Autodesk Inventor part; units mm, degrees
ref_plane "YZ Plane" through (0, 0, 0) normal (1, 0, 0) x (0, 1, 0)
ref_plane "XZ Plane" through (0, 0, 0) normal (0, 1, 0) x (-1, 0, 0)
ref_plane "XY Plane" through (0, 0, 0) normal (0, 0, 1) x (1, 0, 0)
sketch "スケッチ1" plane through (0, 0, 0) normal (0, 0, 1) x (1, 0, 0)
  point P0 (0, 0)
sketch "スケッチ2" plane through (0, 0, 0) normal (0, 0, 1) x (1, 0, 0)
  line L0 (80, -40) -> (-80, -40)
  line L1 (-80, -40) -> (-80, 40)
  line L2 (-80, 40) -> (80, 40)
  line L3 (80, 40) -> (80, -40)
  line L4 (80, -40) -> (-80, 40) construction
  line L5 (-80, -40) -> (80, 40) construction
  circle A0 centre (-48, -19.5) radius 6.05
  circle A1 centre (48, -19.5) radius 12.55
  circle A2 centre (48, -19.5) radius 17.5
  circle A3 centre (65.5, -19.5) radius 2.05
  circle A4 centre (48, -2) radius 2.05
  circle A5 centre (30.5, -19.5) radius 2.05
  circle A6 centre (48, -37) radius 2.05
  circle A7 centre (-48, -19.5) radius 9
  circle A8 centre (-57, -19.5) radius 1.6
  circle A9 centre (-48, -28.5) radius 1.6
  circle A10 centre (-39, -19.5) radius 1.6
  circle A11 centre (-48, -10.5) radius 1.6
  line L6 (75, 35) -> (-75, 35)
  line L7 (-75, 35) -> (-75, -35)
  line L8 (-75, -35) -> (75, -35)
  line L9 (75, -35) -> (75, 35)
  line L10 (-75, 35) -> (-75, 35) construction
  line L11 (-76.6, 35) -> (-76.6, 35)
  line L12 (-73.4, 35) -> (-73.4, 35)
  arc A12 (-73.4, 35) -> (-76.6, 35) centre (-75, 35) ccw
  arc A13 (-76.6, 35) -> (-73.4, 35) centre (-75, 35) ccw
  line L13 (-75, 35) -> (-75, 35) construction
  line L14 (-75, -35) -> (-75, -35) construction
  line L15 (-73.4, -35) -> (-73.4, -35)
  line L16 (-76.6, -35) -> (-76.6, -35)
  arc A14 (-76.6, -35) -> (-73.4, -35) centre (-75, -35) ccw
  arc A15 (-73.4, -35) -> (-76.6, -35) centre (-75, -35) ccw
  line L17 (-75, -35) -> (-75, -35) construction
  line L18 (75, 35) -> (75, 35) construction
  line L19 (73.4, 35) -> (73.4, 35)
  line L20 (76.6, 35) -> (76.6, 35)
  arc A16 (76.6, 35) -> (73.4, 35) centre (75, 35) ccw
  arc A17 (73.4, 35) -> (76.6, 35) centre (75, 35) ccw
  line L21 (75, 35) -> (75, 35) construction
  line L22 (75, -35) -> (75, -35) construction
  line L23 (76.6, -35) -> (76.6, -35)
  line L24 (73.4, -35) -> (73.4, -35)
  arc A18 (73.4, -35) -> (76.6, -35) centre (75, -35) ccw
  arc A19 (76.6, -35) -> (73.4, -35) centre (75, -35) ccw
  line L25 (75, -35) -> (75, -35) construction
  line L26 (-80, -19.5) -> (80, -19.5)
  circle A20 centre (0, -19.5) radius 9
  circle A21 centre (0, -19.5) radius 39
  line L27 (-85, 40) -> (85, 40)
  line L28 (85, 40) -> (85, 35)
  line L29 (85, 35) -> (-85, 35)
  line L30 (-85, 35) -> (-85, 40)
  line L31 (-85, 35) -> (0, 0)
  line L32 (0, 0) -> (85, 35)
  line L33 (-80, 0) -> (80, 0)
  line L34 (80, 0) -> (80, -50)
  line L35 (80, -50) -> (-80, -50)
  line L36 (-80, -50) -> (-80, 0)
  circle A22 centre (-65, 35) radius 1.6
  circle A23 centre (65, 35) radius 1.6
  circle A24 centre (-65, -35) radius 1.6
  circle A25 centre (65, -35) radius 1.6
  point P0 (-75, 35)
  point P1 (-75, -35)
  point P2 (75, 35)
  point P3 (75, -35)
  point P4 (-39.1422, -21.0937)
  point P5 (-39.1422, -17.9063)
  point P6 (0, 40)
  point P7 (85, 40)
  point P8 (48.45, -35)
  point P9 (47.55, -35)
  point P10 (80, 40)
  point P11 (80, 32.9412)
  point P12 (-80, 32.9412)
  point P13 (-80, 40)
  point P14 (60, -23.1746)
  point P15 (60, -15.8254)
  point P16 (0, 35)
  point P17 (-73.4, -35)
  point P18 (-76.6, -35)
  point P19 (73.4, -35)
  point P20 (76.6, -35)
  point P21 (76.6, 35)
  point P22 (73.4, 35)
  point P23 (-76.6, 35)
  point P24 (-73.4, 35)
  dimension "d9" = 35
  dimension "d15" = 18
  dimension "d0" = 160
  dimension "d1" = 80
  dimension "d5" = 12.1
  dimension "d6" = 25.1
  dimension "d10" = 4.1
  dimension "d13" = 360
  dimension "d16" = 3.2
  dimension "d19" = 360
  dimension "d21" = 5
  dimension "d22" = 0
  dimension "d23" = 90
  dimension "d24" = 3.2
  dimension "d25" = 0
  dimension "d26" = 90
  dimension "d27" = 3.2
  dimension "d28" = 0
  dimension "d29" = 90
  dimension "d30" = 3.2
  dimension "d31" = 0
  dimension "d32" = 90
  dimension "d33" = 3.2
  dimension "d36" = 20.5
  dimension "d37" = 18
  dimension "d38" = 78
  dimension "d39" = 48
  dimension "d40" = 48
  dimension "d43" = 170
  dimension "d44" = 85
  dimension "d46" = 50
  dimension "d47" = 3.2
  dimension "d48" = 3.2
  dimension "d51" = 130
  dimension "d52" = 65
extrude "押し出し1" add sketch "スケッチ2" along normal blind 3 contours L0 A21 L8 A2 A6 A25 A18 A19 L9 L26 L3 | L0 A21 L8 | L26 L9 L33 L3 | L0 L1 L26 L7 A15 A14 L8 A24 A21 | A21 A2 L8 | L8 A21 A10 L26 A20 A5 A2 | L33 L9 L32 L3 | L26 A3 A2 A4 L33 L9 | L9 A19 L8 A25 A2 A3 L26 | L8 A24 A15 L7 L26 A8 A7 A9 A10 A21 | L8 A6 A2 | A2 A21 A1 L26 A3 L8 A6 | A2 A5 L26 A1 A21 | L32 L9 A17 L29 L3 | L33 A4 A21 L32 L9 | L26 A2 A3 | A3 A2 L26 | L1 L33 L7 L26 | A21 L26 A10 | A10 A7 A21 | A6 L8 A2 | A2 A6 | A6 L8 | A5 L26 A2 | A2 L26 A5 | A21 L26 A1 | A1 L26 A21 | L29 A16 L6 A23 A22 A12 L1 L2 L3 | L32 A21 L31 L7 A13 L6 A22 A23 A17 L9 | L33 A4 | A4 A2 L33 | A3 L26 A1 A21 A2 A4 | A2 L26 A3 | A3 L26 A2 | L1 L31 L7 L33 | L7 L33 A21 A10 A7 A11 A8 L26 | A10 L26 A7 | A7 A9 A8 L26 A0 A10 | L26 A21 A10 | A10 A21 L33 A2 A5 L26 A20 | L26 A10 A7 | A7 A10 A21 | A6 L8 A2 | L26 A5 A2 | A2 A5 L26 | A5 A2 A21 A1 L26 | A1 A21 L26 | L26 A21 A1 | L32 L31 A21 | A21 L33 L32 | A4 A2 A21 L33 | A4 A2 | L1 L29 A13 L7 L31 | L7 L31 A21 L33 | L26 A7 A8 | A8 A7 L26 | A9 A7 | A7 A9 | L26 A0 A8 A7 A11 A10 | L31 L33 A21 | A8 L26 A7 | A7 L26 A8 | L26 A0 | A0 L26 | A11 A7 | A7 A11
fillet "フィレット1" radius 4 2 edges at (80, 40, 1.5) (-80, 40, 1.5)
equation "\"d27\" = d24"
equation "\"d30\" = d24"
equation "\"d33\" = d24"
equation "\"d40\" = d39"
properties part number "aaa_small_plate_no"
CAD build for the part. Positions are in the model's coordinates, mm. Give positions to 0.01 mm unless a question says otherwise; leave off trailing zeros. Order: outer loops, then holes, each group sorted by start corner. A loop starts at its lowest first (then second) coordinate and runs counter-clockwise, first axis right, second up.
(1) Mould opens along X. For faces 1 (the cylindrical face through (-78.797, 38.859, 1.521)), 2 (the flat face through (80, -1, 1)), 3 (the cylindrical face through (-63.52, 35.61, 1.48)) say: released by +X, released by -X, zero draft, split by the parting line, or undercut.
(2) Flat gauge pins, fed straight in: pin 1 (10 mm diameter, centred on x = -26.5, y = -1, fed in from -Z); pin 2 (1.9 mm diameter, centred on x = 65, y = 35, fed in from +Z). Where does each tip first touch, or does it go through?
(3) Saw through at A-A, the plane x = 65. Give the cut face in (y, z).
(4) Drill centre lines: L1, parallel to Y at x = 65, z = 0.6; L2, parallel to X at y = 35, z = 1.55; L3, parallel to X at y = -19.5, z = 0.9. Where is each one in solid material? Low to high.
(5) Saw through at D-D, the plane y = -13. Give the cut face in (x, z), then the cut area to 3 significant figures.
(6) Saw through at B-B, the plane y = -35. Give the cut face in (x, z).
(7) Saw through at C-C, the plane z = 2.1. State how many separate pieces and enclosed holes the cut face has, then the cut area to 3 significant figures.
Results found:
1. face 1: released by -X
1. face 2: released by +X
1. face 3: undercut
2. pin 1: stops at z = 0
2. pin 2: passes through
3. outline: (-40, 0) - (-36.6, 0) - (-36.6, 3) - (-40, 3) - close; (-33.4, 0) - (33.4, 0) - (33.4, 3) - (-33.4, 3) - close; (36.6, 0) - (40, 0) - (40, 3) - (36.6, 3) - close
4. L1: y = -40 to -36.6, -33.4 to 33.4, 36.6 to 40
4. L2: x = -80 to -76.6, -73.4 to -66.6, -63.4 to 63.4, 66.6 to 73.4, 76.6 to 80
4. L3: x = -80 to -9, 9 to 80
5. outline: (-80, 0) - (-6.22, 0) - (-6.22, 3) - (-80, 3) - close; (6.22, 0) - (80, 0) - (80, 3) - (6.22, 3) - close
5. area: 443 mm2
6. outline: (-80, 0) - (-76.6, 0) - (-76.6, 3) - (-80, 3) - close; (-73.4, 0) - (-66.6, 0) - (-66.6, 3) - (-73.4, 3) - close; (-63.4, 0) - (63.4, 0) - (63.4, 3) - (-63.4, 3) - close; (66.6, 0) - (73.4, 0) - (73.4, 3) - (66.6, 3) - close; (76.6, 0) - (80, 0) - (80, 3) - (76.6, 3) - close
7. separate pieces: 1
7. enclosed holes: 9
7. area: 12,500 mm2
